```python
from build123d import *

# Parameters (mm, degrees)
SKETCH1_R           = 70
SKETCH1_R_2         = 4.5
BOSS_EXTRUDE1_DEPTH = 16
CUT_EXTRUDE1_START  = -4
SKETCH2_R           = 70
SKETCH2_R_2         = 45
CUT_EXTRUDE1_DEPTH  = 4
SKETCH3_R           = 40
CUT_EXTRUDE2_DEPTH  = 2
SKETCH4_R           = 25.25
CUT_EXTRUDE3_DEPTH  = 24
SKETCH7_R           = 35
CUT_EXTRUDE5_DEPTH  = 10


with BuildPart() as part:
    # Sketch1 → Boss-Extrude1 (new body)
    with BuildSketch(Plane.XY):
        Circle(SKETCH1_R)
        with Locations((0, 57.5)):
            Circle(SKETCH1_R_2, mode=Mode.SUBTRACT)
        with Locations((57.5, 0)):
            Circle(SKETCH1_R_2, mode=Mode.SUBTRACT)
        with Locations((0, -57.5)):
            Circle(SKETCH1_R_2, mode=Mode.SUBTRACT)
        with Locations((-57.5, 0)):
            Circle(SKETCH1_R_2, mode=Mode.SUBTRACT)
    extrude(amount=BOSS_EXTRUDE1_DEPTH)

    # Sketch2 → Cut-Extrude1 (cut)
    with BuildSketch(Plane.XY.offset(16).offset(CUT_EXTRUDE1_START)):
        Circle(SKETCH2_R)
        Circle(SKETCH2_R_2, mode=Mode.SUBTRACT)
    extrude(amount=CUT_EXTRUDE1_DEPTH, mode=Mode.SUBTRACT)

    # Sketch3 → Cut-Extrude2 (cut)
    with BuildSketch(Plane.XY.offset(16)):
        Circle(SKETCH3_R)
    extrude(amount=-CUT_EXTRUDE2_DEPTH, mode=Mode.SUBTRACT)

    # Sketch4 → Cut-Extrude3 (cut)
    with BuildSketch(Plane.XY.offset(14)):
        Circle(SKETCH4_R)
    extrude(amount=-CUT_EXTRUDE3_DEPTH, mode=Mode.SUBTRACT)

    # Sketch7 → Cut-Extrude5 (cut)
    with BuildSketch(Plane.XY.offset(14)):
        Circle(SKETCH7_R)
    extrude(amount=-CUT_EXTRUDE5_DEPTH, mode=Mode.SUBTRACT)


solid = part.part
```
Can you work these out from the model? Positions are in its coordinate system, mm. A direction names the side the tool comes from. Round coordinates to 2 decimals unless told otherwise and drop trailing zeros. Loops run counter-clockwise (first coordinate to the right, second up) from the corner with the lowest first, then second, coordinate; pieces in that order, holes last. Notation, with made-up numbers: (85.5, 12.25) -> (114.5, 12.25) arc R28 cw to (114.5, 39.25) -> close; hole circle Ø3 at (23.25, 35.25). An arc over 180 degrees is marked (long way). Answer in a Markdown table with one row per item.
Item 1: If I drill on probe 1 along X at (y, z) = (-14, 12.75); probe 2 along Y at (x, z) = (-57.5, 7.25); probe 3 along X at (y, z) = (13.5, 1.75), over which ranges is the centre line in solid material (lowest first)?
Answer block:
| item | result |
|---|---|
| probe 1 | -42.77 to -32.08, 32.08 to 42.77 |
| probe 2 | -39.92 to -4.5, 4.5 to 39.92 |
| probe 3 | -68.69 to -21.34, 21.34 to 68.69 |
Item 2: Suppose I cut it at D-D, the plane y = -57.5. List the corners of the cut face in (x, z) for me.
Answer block:
| item | result |
|---|---|
| outline | (-39.92, 0) -> (-4.5, 0) -> (-4.5, 12) -> (-39.92, 12) -> close; (4.5, 0) -> (39.92, 0) -> (39.92, 12) -> (4.5, 12) -> close |
Item 3: Suppose I cut it at A-A, the plane y = 0. List the corners of the cut face in (x, z) for me.
Answer block:
| item | result |
|---|---|
| outline | (-70, 0) -> (-62, 0) -> (-62, 12) -> (-70, 12) -> close; (-53, 0) -> (-25.25, 0) -> (-25.25, 4) -> (-35, 4) -> (-35, 14) -> (-40, 14) -> (-40, 16) -> (-45, 16) -> (-45, 12) -> (-53, 12) -> close; (25.25, 0) -> (53, 0) -> (53, 12) -> (45, 12) -> (45, 16) -> (40, 16) -> (40, 14) -> (35, 14) -> (35, 4) -> (25.25, 4) -> close; (62, 0) -> (70, 0) -> (70, 12) -> (62, 12) -> close |
Item 4: Suppose I cut it at C-C, the plane z = 6.25. List the corners of the cut face in (x, y) for me.
Answer block:
| item | result |
|---|---|
| outline | circle Ø140 at (0, 0); hole circle Ø9 at (-57.5, 0); hole circle Ø70 at (0, 0); hole circle Ø9 at (0, -57.5); hole circle Ø9 at (0, 57.5); hole circle Ø9 at (57.5, 0) |
Item 5: On a 3-axis mill with a long thin cutter (end or side, diameter ignored), from which of +Z, -Z, +X, -X, +Y, -Y can I reach the whole of each face in a straight line? I mean faces 1 (the cylindrical face through (-8.67, -39.05, 15.01)), 2 (the cylindrical face through (-55.55, -42.594, 5.916)). Say none if no direction works.
Answer block:
| item | result |
|---|---|
| face 1 | +Z |
| face 2 | +Z, -Z |
Item 6: We'd pull the mould along X, two halves only. Please class faces 3 (the flat face through (-1, -30, 0)), 4 (the cylindrical face through (20.765, -39.923, 13.972)), 5 (the cylindrical face through (-28, -21, 9)), 6 (the cylindrical face through (-5.47, -24.65, 2.03)): released by +X, released by -X, zero draft, split by the parting line, or undercut.
Answer block:
| item | result |
|---|---|
| face 3 | zero draft |
| face 4 | split by the parting line |
| face 5 | undercut |
| face 6 | undercut |
Item 7: Will these pins go through, and if not, where does the flat tip stop? P1, Ø6, axis at y = 37.5, z = 2, coming from the +X side; P2, Ø1.5, axis at y = 12, z = 10, coming from the -X side; P3, Ø2, axis at y = 37, z = 11, coming from the -X side; P4, Ø1, axis at x = 2.5, y = -31, coming from the -Z side.
Answer block:
| item | result |
|---|---|
| P1 | x = 60.91 |
| P2 | x = -69.09 |
| P3 | x = -60.03 |
| P4 | z = 0 |
